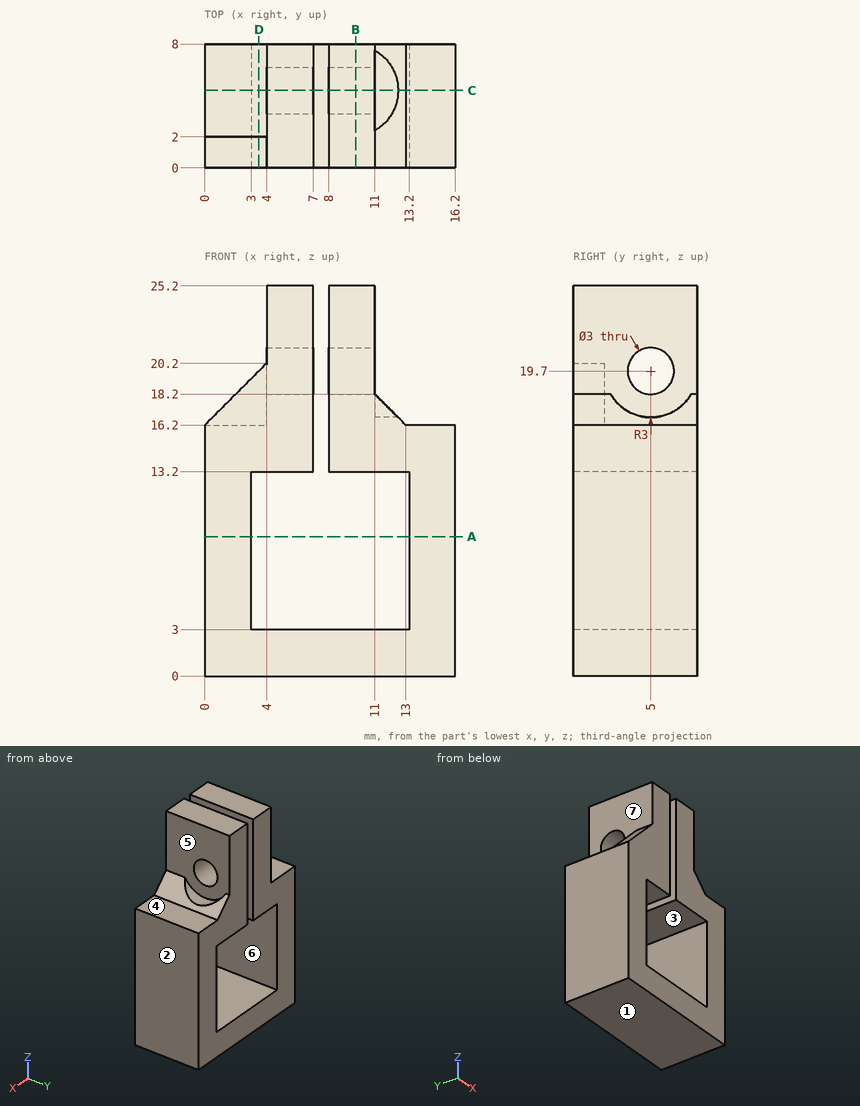
Verification items for this drawing (mm, ordinates from the low corner). A direction names the side the tool comes from. Give positions to 0.01 mm unless a question says otherwise; leave off trailing zeros. Write each loop counter-clockwise with the first axis right and the second up, starting at its lowest first coordinate (ties: lowest second). Pieces come first, ordered by that corner, then holes. Notation, with made-up numbers: (66.5, 65.5) -> (91.5, 65.5) arc R32 ccw to (91.5, 97.5) -> close; hole circle Ø9 at (2.5, 70). An arc over 180 degrees is marked (long way). Write item = value, one per line.
Item 1: Sectioned sample at B-B on x = 9.75. Record the boundary of the cut face in (y, z), and give its area (3 significant figures).
Output:
outline = (0, 0) -> (8, 0) -> (8, 3) -> (0, 3) -> close; (0, 13.2) -> (8, 13.2) -> (8, 25.2) -> (0, 25.2) -> close; hole circle Ø3 at (5, 19.7)
area = 113 mm^2
Item 2: Release check for a two-part mould opening along X. For the marked faces 1, 2 and 3 record: +X half, -X half, draft (parallel to the pull), parting line (faces both ways), or undercut.
Output:
face_1 = draft
face_2 = +X half
face_3 = undercut
Item 3: Sectioned sample at D-D on x = 3.5. Record the boundary of the cut face in (y, z).
Output:
outline = (0, 0) -> (8, 0) -> (8, 3) -> (0, 3) -> close; (0, 13.2) -> (8, 13.2) -> (8, 16.2) -> (2, 16.2) -> (2, 19.7) -> (0, 19.7) -> close
Item 4: Gauge pin test, flat ends, axial feed: pin 1 (4 mm diameter, centred on y = 2.5, z = 22, fed in from -X); pin 2 (3 mm diameter, centred on x = 4, y = 1.5, fed in from -Z); pin 3 (1.2 mm diameter, centred on x = 2.5, y = 6, fed in from +Z); pin 4 (4 mm diameter, centred on y = 3, z = 19.5, fed in from +X). Record the tip position at first contact, or that the pin passes through.
Output:
pin_1 = 3.86
pin_2 = 0
pin_3 = 16.2
pin_4 = 11.7
Item 5: Tool access check on the marked faces 4, 5, 6 and 7. Record the directions out of +Z, -Z, +X, -X, +Y, -Y that give a thin tool (end or side, any length) a straight path to the whole face; none if there is none.
Output:
face_4 = +Z, +X, +Y, -Y
face_5 = +Z, +X
face_6 = +Y, -Y
face_7 = +Z, -X, +Y
Item 6: Scan lines: probe 1 along Z at (x, y) = (6.25, 5); probe 2 along X at (y, z) = (3.25, 10.75); probe 3 along X at (y, z) = (2.5, 23). Record each from-to range of solid material in increasing order. Write a range as from..to.
Output:
probe_1 = 0..3, 13.2..18.2, 21.2..25.2
probe_2 = 0..3, 13.2..16.2
probe_3 = 4..7, 8..11
Item 7: Sectioned sample at A-A on z = 9. Record the boundary of the cut face in (x, y).
Output:
outline = (0, 0) -> (3, 0) -> (3, 8) -> (0, 8) -> close; (13.2, 0) -> (16.2, 0) -> (16.2, 8) -> (13.2, 8) -> close
Item 8: Sectioned sample at C-C on y = 5. Record the boundary of the cut face in (x, z).
Output:
outline = (0, 0) -> (16.2, 0) -> (16.2, 16.2) -> (13, 16.2) -> (12.5, 16.7) -> (11, 16.7) -> (11, 18.2) -> (8, 18.2) -> (8, 13.2) -> (13.2, 13.2) -> (13.2, 3) -> (3, 3) -> (3, 13.2) -> (7, 13.2) -> (7, 18.2) -> (4, 18.2) -> (4, 16.2) -> (0, 16.2) -> close; (4, 21.2) -> (7, 21.2) -> (7, 25.2) -> (4, 25.2) -> close; (8, 21.2) -> (11, 21.2) -> (11, 25.2) -> (8, 25.2) -> close
